```python
from build123d import *

# Parameters (mm, degrees)
F0_R     = 2.5
F1_DEPTH = 2
F2_R     = 6
F2_R_2   = 2.5
F3_DEPTH = 9
F4_R     = 2
F5_R     = 1.99999


# Not quite as in the source:
# - a fillet or chamfer is up to 0.001 mm smaller than in the source, because OpenCascade refuses the exact size


with BuildPart() as f1:
    # F0 (on Top) → F1 (new body)
    with BuildSketch(Plane.XY):
        with BuildLine():
            Line((-30, -5), (-7.4833147735, -5))
            ThreePointArc((-7.4833147735, -5), (-6.3639610307, -6.3639610307), (-5, -7.4833147735))
            Line((-5, -7.4833147735), (-5, -15))
            ThreePointArc((-5, -15), (0, -20), (5, -15))
            Line((5, -15), (5, -7.4833147735))
            ThreePointArc((5, -7.4833147735), (6.3639610307, -6.3639610307), (7.4833147735, -5))
            Line((7.4833147735, -5), (30, -5))
            ThreePointArc((30, -5), (35, 0), (30, 5))
            Line((30, 5), (7.4833147735, 5))
            ThreePointArc((7.4833147735, 5), (6.3639610307, 6.3639610307), (5, 7.4833147735))
            Line((5, 7.4833147735), (5, 15))
            ThreePointArc((5, 15), (0, 20), (-5, 15))
            Line((-5, 15), (-5, 7.4833147735))
            ThreePointArc((-5, 7.4833147735), (-6.3639610307, 6.3639610307), (-7.4833147735, 5))
            Line((-7.4833147735, 5), (-30, 5))
            ThreePointArc((-30, 5), (-35, 0), (-30, -5))
        make_face()
        Circle(F0_R, mode=Mode.SUBTRACT)
    extrude(amount=F1_DEPTH)

    # F2 (on face) → F3 (join)
    with BuildSketch(Plane.XY.offset(2)):
        Circle(F2_R)
        Circle(F2_R_2, mode=Mode.SUBTRACT)
    extrude(amount=F3_DEPTH)

    # F4
    f4_edges = [f1.edges().sort_by_distance(p)[0] for p in [
        (-6, 0, 11),
    ]]
    fillet(f4_edges, radius=F4_R)

    # F5 (radius 2 in the source; OpenCascade refuses exactly that, so slightly less here)
    f5_edges = [f1.edges().sort_by_distance(p)[0] for p in [
        (35, 0, 2),
        (0, 20, 2),
        (0, -20, 2),
        (-35, 0, 2),
    ]]
    fillet(f5_edges, radius=F5_R)


solid = f1.part
```
CAD build for the part. Positions are in the model's coordinates, mm. A direction names the side the tool comes from. Round coordinates to 2 decimals unless told otherwise and drop trailing zeros. Order: outer loops, then holes, each group sorted by start corner. A loop starts at its lowest first (then second) coordinate and runs counter-clockwise, first axis right, second up. Notation, with made-up numbers: (45.5, 29) - (72.5, 29) arc R8 ccw to (72.5, 35) - close; hole circle Ø2 at (22.25, -8). An arc over 180 degrees is marked (long way). Answer as CSV lines item,"result". Start each with the question number.
1. Drill centre lines: L1, parallel to Y at x = 0, z = 5; L2, parallel to Z at x = 0, y = -11; L3, parallel to Z at x = 0.5, y = 5. Where is each one in solid material? Low to high. Write a range as [from, to].
2. Pin check, flat tips, straight feed: pin 1 (5 mm diameter, centred on x = 0, y = -5.5, fed in from -Z); pin 2 (4 mm diameter, centred on x = -3.5, y = -11, fed in from +Z). Stop position of each tip, or through.
3. Tool access for faces 5 (the face through (6.404, 6.324, 0.986)), 6 (the face through (-18.58, -4.4, 1.43)), 7 (the face through (4.4, -11.19, 1.43)), 8 (the face through (-18.9, 4.4, 1.43)): list every direction of +Z, -Z, +X, -X, +Y, -Y with a clear straight run to the whole face (end or side of a thin tool).
4. Saw through at C-C, the plane z = 7.75. Write the cut outline in (x, y).
5. Pull direction X, two halves, no side cores. Call faces 1 (the face through (-4.4, -11.29, 1.43)), 2 (the face through (18.58, 4.4, 1.43)), 3 (the face through (-0.54, -2.44, 5.42)), 4 (the face through (-6, 0, 5)): +X half, -X half, draft (parallel to the pull), parting line (faces both ways), or undercut.
Model answer:
1,L1,"y = [-6, -2.5], [2.5, 6]"
1,L2,"z = [0, 2]"
1,L3,"z = [0, 10.72]"
2,pin 1,"stops at z = 0"
2,pin 2,"stops at z = 2"
3,face 5,"+Z, +X, +Y"
3,face 6,"+Z, -X, -Y"
3,face 7,"+Z, +X, -Y"
3,face 8,"+Z, -X, +Y"
4,outline,"circle Ø12 at (0, 0); hole circle Ø5 at (0, 0)"
5,face 1,"-X half"
5,face 2,"draft"
5,face 3,"undercut"
5,face 4,"parting line"
